Solid Edge part; units mm, degrees
sketch "Sketch1" plane through (0, 0, 0) normal (0, -1, 0) x (1, 0, 0)
  line L0 (21, 16.97) -> (16.97, 21)
  line L1 (16.97, 21) -> (-16.97, 21)
  line L2 (-16.97, 21) -> (-21, 16.97)
  line L3 (-21, 16.97) -> (-21, -16.97)
  line L4 (-21, -16.97) -> (-16.97, -21)
  line L5 (-16.97, -21) -> (16.97, -21)
  line L6 (16.97, -21) -> (21, -16.97)
  line L7 (21, -16.97) -> (21, 16.97)
  line L8 (26, 19.0411) -> (19.0411, 26)
  line L9 (19.0411, 26) -> (-19.0411, 26)
  line L10 (-19.0411, 26) -> (-26, 19.0411)
  line L11 (-26, 19.0411) -> (-26, -19.0411)
  line L12 (-26, -19.0411) -> (-19.0411, -26)
  line L13 (-19.0411, -26) -> (19.0411, -26)
  line L14 (19.0411, -26) -> (26, -19.0411)
  line L15 (26, -19.0411) -> (26, 19.0411)
extrude "Protrusion1" add sketch "Sketch1" against normal blind 35
sketch "Sketch2" plane through (0, 0, 0) normal (0, -1, 0) x (1, 0, 0)
  line L0 (19.0411, 26) -> (-19.0411, 26)
  line L1 (-19.0411, 26) -> (-26, 19.0411)
  line L2 (-26, 19.0411) -> (-26, -19.0411)
  line L3 (-26, -19.0411) -> (-19.0411, -26)
  line L4 (-19.0411, -26) -> (19.0411, -26)
  line L5 (19.0411, -26) -> (26, -19.0411)
  line L6 (26, -19.0411) -> (26, 19.0411)
  line L7 (26, 19.0411) -> (19.0411, 26)
extrude "Deckel" add sketch "Sketch2" along normal blind 5
hole "Motorwelle" at (0, -5, 0) direction (0, 1, 0) diameter 6 end up to next
hole "Hole1" at (-15.5, -5, -15.5) direction (0, 1, 0) diameter 3.2 end up to next start chamfer 0.2 start chamfer angle 45
hole "Hole2" at (-15.5, -5, 15.5) direction (0, 1, 0) diameter 3.2 end up to next start chamfer 0.2 start chamfer angle 45
hole "Hole3" at (15.5, -5, 15.5) direction (0, 1, 0) diameter 3.2 end up to next start chamfer 0.2 start chamfer angle 45
hole "Hole4" at (15.5, -5, -15.5) direction (0, 1, 0) diameter 3.2 end up to next start chamfer 0.2 start chamfer angle 45
sketch "Sketch3" plane through (0, 0, 0) normal (0, 1, 0) x (0, 0, 1)
  circle A0 centre (0, 0) radius 11.5
extrude "Motoflansch" cut sketch "Sketch3" against normal blind 1
sketch "Sketch4" plane through (0, -5, 0) normal (0, -1, 0) x (1, 0, 0)
  line L0 (-26, 19.0411) -> (-19.0411, 26)
  line L1 (-19.0411, 26) -> (4, 26)
  line L2 (4, 26) -> (4, 56)
  line L3 (-26, 56) -> (4, 56)
  line L4 (-26, 19.0411) -> (-26, 56)
  dimension "D1" = 4
  dimension "D2" = 26
extrude "Motoraufhängung_Leiste" add sketch "Sketch4" against normal blind 23
sketch "Sketch5" plane through (-13, 18, 33.5205) normal (0, 1, 0) x (-1, 0, 0)
  line L0 (-17, -7.5205) -> (-17, 22.4795)
  line L1 (-17, 22.4795) -> (-12, 22.4795)
  line L2 (-12, 22.4795) -> (-12, -7.5205)
  line L3 (-12, -7.5205) -> (-17, -7.5205)
  dimension "D1" = 17
extrude "Zentrierung_Leiste" add sketch "Sketch5" along normal blind 17.5
sketch "Sketch6" plane through (0, -5, 11) normal (0, -1, 0) x (1, 0, 0)
  line L0 (-26, -30.0411) -> (-26, 8.0411)
  line L1 (-26, 8.0411) -> (-63, 8.0411)
  line L2 (-66, 5.0411) -> (-63, 8.0411)
  line L3 (-66, 5.0411) -> (-66, -27.0411)
  line L4 (-63, -30.0411) -> (-66, -27.0411)
  line L5 (-63, -30.0411) -> (-26, -30.0411)
  dimension "D1" = 63
  dimension "D2" = 66
  dimension "D3" = 66
extrude "Auflage_auf_Platte" add sketch "Sketch6" against normal blind 23
hole "Bohrung_Alustange" at (-11, 5, 56) direction (0, 0, -1) diameter 8 depth 11 tip angle 118 start chamfer 0.2 start chamfer angle 45
sketch "Sketch7" plane through (0, 35, 0) normal (0, 1, 0) x (1, 0, 0)
  line L0 (-19.0411, 26) -> (-16.97, 21)
  line L1 (-16.97, 21) -> (-16.97, -21)
  line L2 (-16.97, -21) -> (-19.0411, -26)
  line L3 (-19.0411, -26) -> (-26, -26)
  line L4 (-26, -26) -> (-26, 26)
  line L5 (-26, 26) -> (-19.0411, 26)
extrude "Motorseite" cut sketch "Sketch7" against normal blind 17
hole "Hole5" at (-8, -5, 32) direction (0, 1, 0) diameter 4.3 end up to next
hole "Hole6" at (-15, -5, 41) direction (0, 1, 0) diameter 4.3 end up to next
hole "Hole7" at (-59, -5, 12.0411) direction (0, 1, 0) diameter 4.3 end up to next
hole "Hole8" at (-59, -5, -12.0411) direction (0, 1, 0) diameter 4.3 end up to next
hole "Hole9" at (-46, -5, 0) direction (0, 1, 0) diameter 4.3 end up to next
fillet "Verrundung_Innen" radius 3 3 edges at (-26, 6.5, -19.0411) (-26, 6.5, 19.0411) (4, 15, 26)
fillet "Verrundung_spitzeEcke" radius 5 2 edges at (-19.0411, 26.5, 26) (-19.0411, 26.5, -26)
sketch "Sketch8" plane through (4.515, 35, 1.5) normal (0, 1, 0) x (0, 0, -1)
  line L0 (-15.5321, 25.665) -> (18.5321, 25.665)
  line L1 (18.5321, 25.665) -> (22.65, 21.5471)
  line L2 (22.65, 21.5471) -> (22.65, -12.5171)
  line L3 (22.65, -12.5171) -> (18.5321, -16.635)
  line L4 (18.5321, -16.635) -> (-15.5321, -16.635)
  line L5 (-15.5321, -16.635) -> (-19.65, -12.5171)
  line L6 (-19.65, -12.5171) -> (-19.65, 21.5471)
  line L7 (-19.65, 21.5471) -> (-15.5321, 25.665)
extrude "Verbreiterung" cut sketch "Sketch8" against normal blind 35
Build history of the part. All positions in model axes, mm. A direction names the side the tool comes from. Give positions to 0.01 mm unless a question says otherwise; leave off trailing zeros. Loops run counter-clockwise (first coordinate to the right, second up) from the corner with the lowest first, then second, coordinate; pieces in that order, holes last.
1) 3-axis set-ups, long thin cutter, end or side, ignore diameter. For faces 1 (the face through (0, 18, 21.15)), 2 (the face through (-14.966, 5.521, 50.324)), 3 (the face through (16.58, -2.43, 16.68)), 4 (the face through (2, 35.5, 41)), 5 (the face through (13, 15, 26)): which of +Z, -Z, +X, -X, +Y, -Y reach the whole face in a straight line?
Values follow:
face 1: +Y
face 2: +Z
face 3: +Y, -Y
face 4: +Z, -Z, +X, -X, +Y
face 5: +Z, +X, +Y, -Y
2) Band-saw the part on C-C on z = 51.5. List the corners of the cut face in (x, y), then the cut area to 3 significant figures.
Values follow:
outline: (-26, -5) - (4, -5) - (4, 35.5) - (-1, 35.5) - (-1, 18) - (-26, 18) - close; hole circle Ø8 at (-11, 5)
area: 727 mm2
3) Band-saw the part on D-D on x = -46. List the corners of the cut face in (y, z), then the cut area to 3 significant figures.
Values follow:
outline: (-5, -19.04) - (18, -19.04) - (18, -2.15) - (-5, -2.15) - close; (-5, 2.15) - (18, 2.15) - (18, 19.04) - (-5, 19.04) - close
area: 777 mm2
4) Drop flat-ended pins along their axis: P1, Ø11.5, axis at x = -37, y = 9.5, coming from the -Z side; P2, Ø1, axis at x = -33, y = 16, coming from the +Z side; P3, Ø2, axis at x = -36, z = 17, coming from the +Y side; P4, Ø5, axis at x = -13.5, y = 19, coming from the -Z side. Give the stop position or say it passes through.
Values follow:
P1: stops at z = -19.04
P2: stops at z = 19.04
P3: stops at y = 18
P4: stops at z = -26
5) Probe line 1 along X through (y, z) = (-2.65, 0); line 2 along X through (y, z) = (-1.2, 15.5); line 3 along Z through (x, y) = (-3, 13). List the from-to ranges inside material, lowest first.
Values follow:
line 1: x = -66 to -48.15, -43.85 to -3, 3 to 26
line 2: x = -66 to -17.1, -13.9 to 13.9, 17.1 to 26
line 3: z = -26 to -21.15, 21.15 to 56
6) Two-plate mould, pull along Z, no slides. Class faces 6 (the face through (-11, 10, 56)), 7 (the face through (-66, 6, 0)), 8 (the face through (19.06, 17.74, -19.12)): released by +Z, released by -Z, zero draft, split by the parting line, or undercut.
Values follow:
face 6: released by +Z
face 7: zero draft
face 8: undercut
7) Band-saw the part on A-A on z = 32. List the corners of the cut face in (x, y).
Values follow:
outline: (-26, -5) - (-10.15, -5) - (-10.15, 18) - (-26, 18) - close; (-5.85, -5) - (4, -5) - (4, 35.5) - (-1, 35.5) - (-1, 18) - (-5.85, 18) - close
8) Band-saw the part on B-B on x = -59. List the corners of the cut face in (y, z), then the cut area to 3 significant figures.
Values follow:
outline: (-5, -19.04) - (18, -19.04) - (18, -14.19) - (-5, -14.19) - close; (-5, -9.89) - (18, -9.89) - (18, 9.89) - (-5, 9.89) - close; (-5, 14.19) - (18, 14.19) - (18, 19.04) - (-5, 19.04) - close
area: 678 mm2
